Design review of the part built by this model. Coordinates are the model's own, in mm. A direction names the side the tool comes from. Coordinates: 2 decimals unless noted, no trailing zeros. Write each loop counter-clockwise with the first axis right and the second up, starting at its lowest first coordinate (ties: lowest second). Pieces come first, ordered by that corner, then holes. Notation, with made-up numbers: M -8.75,50 L -4.75,50 A23 ccw -4.75,89 Z; hole C 51,-30 d6. An arc over 180 degrees is marked long. One line per question, with ' | ' between items.
from build123d import *

# Parameters (mm, degrees)
SKETCH1_W                           = 184.15
SKETCH1_H                           = 50.8
BOSS_EXTRUDE1_DEPTH                 = 10.16
CUT_EXTRUDE1_DEPTH                  = 110.402922012
CUT_EXTRUDE1_DEPTH_BACK             = 110.402922012
SKETCH7_R                           = 22.847252038
BOSS_EXTRUDE2_DEPTH                 = 50.8
SKETCH8_R                           = 18.9865
CUT_EXTRUDE2_DEPTH                  = 45.72
SKETCH9_R                           = 7.9375
CUT_EXTRUDE3_DEPTH                  = 115.259711281
BOSS_EXTRUDE3_DEPTH                 = 50.8
BOSS_EXTRUDE4_START                 = -50.8
BOSS_EXTRUDE4_DEPTH                 = 50.8
BOSS_EXTRUDE5_START                 = -50.8
BOSS_EXTRUDE5_DEPTH                 = 50.8
CUT_EXTRUDE6_DEPTH                  = 117.385579957
F_10_CLEARANCE_HOLE1_D              = 5.1054
F_10_CLEARANCE_HOLE2_D              = 5.1054
SKETCH31_W                          = 29.960646913
SKETCH31_H                          = 50.8
BOSS_EXTRUDE6_DEPTH                 = 2.54
F_3_16_0_1875_DIAMETER_HOLE3_REACH  = 132.668
F_3_16_0_1875_DIAMETER_HOLE3_BORE_R = 2.38125
F_3_16_0_1875_DIAMETER_HOLE4_REACH  = 129.945
F_3_16_0_1875_DIAMETER_HOLE4_BORE_R = 2.38125


with BuildPart() as part:
    # Sketch1 → Boss-Extrude1 (new body)
    with BuildSketch(Plane.XY):
        with Locations((4.284398839, -3.653036721)):
            Rectangle(SKETCH1_W, SKETCH1_H)
    extrude(amount=BOSS_EXTRUDE1_DEPTH)

    # Sketch6 → Cut-Extrude1 (cut, two sides: drawn at the far end of the back side and taken through both)
    with BuildSketch(Plane(origin=(0, 21.746963279, 0), x_dir=(1, 0, 0), z_dir=(0, 1, 0)).offset(-CUT_EXTRUDE1_DEPTH_BACK)):
        with BuildLine():
            Line((189.051531618, 108.11571126), (10.888398839, 0))
            ThreePointArc((10.888398839, 0), (4.284398839, -1.847030056), (-2.319601161, 0))
            Line((-2.319601161, 0), (-180.48273394, 108.11571126))
            Line((-180.48273394, 108.11571126), (-180.48273394, 524.918345142))
            Line((-180.48273394, 524.918345142), (189.051531618, 524.918345142))
            Line((189.051531618, 524.918345142), (189.051531618, 108.11571126))
        make_face()
    extrude(amount=CUT_EXTRUDE1_DEPTH + CUT_EXTRUDE1_DEPTH_BACK, mode=Mode.SUBTRACT)

    # Sketch7 → Boss-Extrude2 (add, through all)
    with BuildSketch(Plane(origin=(0, 21.746963279, 0), x_dir=(1, 0, 0), z_dir=(0, 1, 0))):
        with Locations((4.284398839, 18.138470809)):
            Circle(SKETCH7_R)
    extrude(amount=-BOSS_EXTRUDE2_DEPTH)

    # Sketch8 → Cut-Extrude2 (cut)
    with BuildSketch(Plane(origin=(0, 21.746963279, 0), x_dir=(1, 0, 0), z_dir=(0, 1, 0))):
        with Locations(Location((4.284398839, 18.138470809, 0), (0, 0, 270))):
            Circle(SKETCH8_R)
    extrude(amount=-CUT_EXTRUDE2_DEPTH, mode=Mode.SUBTRACT)

    # Sketch9 → Cut-Extrude3 (cut, through all)
    with BuildSketch(Plane(origin=(0, -23.973036721, 0), x_dir=(1, 0, 0), z_dir=(0, 1, 0))):
        with Locations(Location((4.284398839, 18.138470809, 0), (0, 0, 270))):
            Circle(SKETCH9_R)
    extrude(amount=-CUT_EXTRUDE3_DEPTH, mode=Mode.SUBTRACT)

    # Sketch12 → Boss-Extrude3 (add)
    with BuildSketch(Plane(origin=(0, 21.746963279, 0), x_dir=(1, 0, 0), z_dir=(0, 1, 0))):
        with BuildLine():
            Line((27.131650877, 18.138470763), (27.131650877, 0))
            Line((27.131650877, 0), (18.176583779, 0))
            ThreePointArc((18.176583779, 0), (24.770920949, 8.024157287), (27.131650877, 18.138470763))
        make_face()
        with BuildLine():
            Line((-18.562853199, 18.138470775), (-18.562853199, 0))
            Line((-18.562853199, 0), (-9.607786101, 0))
            ThreePointArc((-9.607786101, 0), (-16.202123271, 8.024157294), (-18.562853199, 18.138470775))
        make_face()
    extrude(amount=-BOSS_EXTRUDE3_DEPTH)

    # Sketch16 → Boss-Extrude4 (add)
    with BuildSketch(Plane.XZ.offset(29.053036721).offset(BOSS_EXTRUDE4_START)):
        with BuildLine():
            Line((-18.562853199, -18.138470775), (-18.562853199, -40.985722847))
            Line((-18.562853199, -40.985722847), (4.284398845, -40.985722847))
            ThreePointArc((4.284398845, -40.985722847), (-11.871048017, -34.293917645), (-18.562853199, -18.138470775))
        make_face()
    extrude(amount=BOSS_EXTRUDE4_DEPTH)

    # Sketch18 → Boss-Extrude5 (add)
    with BuildSketch(Plane.XZ.offset(29.053036721).offset(BOSS_EXTRUDE5_START)):
        with BuildLine():
            Line((27.131650877, -18.138470763), (27.131650877, -40.985722847))
            Line((27.131650877, -40.985722847), (4.284398839, -40.985722847))
            ThreePointArc((4.284398839, -40.985722847), (20.439845703, -34.29391764), (27.131650877, -18.138470763))
        make_face()
    extrude(amount=BOSS_EXTRUDE5_DEPTH)

    # Sketch19 → Cut-Extrude6 (cut, through all)
    with BuildSketch(Plane(origin=(0, 21.746963279, 0), x_dir=(1, 0, 0), z_dir=(0, 1, 0))):
        Polygon((19.257650877, 40.985722847), (27.131650877, 40.985722847), (27.131650877, 33.111722847), align=None)
        Polygon((-18.562853199, 40.985722847), (-18.562853199, 33.125865684), (-10.702996036, 40.985722847), align=None)
    extrude(amount=-CUT_EXTRUDE6_DEPTH, mode=Mode.SUBTRACT)

    # #10 Clearance Hole1 (through all)
    with Locations(Plane(origin=(0, 0, 0), x_dir=(-1, 0, 0), z_dir=(0, 0, -1))):
        with Locations((78.265601161, 9.046963279), (78.265601161, -16.353036721), (-86.834398839, -16.353036721), (-86.834398839, 9.046963279)):
            Hole(F_10_CLEARANCE_HOLE1_D / 2)

    # #10 Clearance Hole2 (through all)
    with Locations(Plane(origin=(0, 0, 0), x_dir=(-1, 0, 0), z_dir=(0, 0, -1))):
        with Locations((27.465601161, -16.353036721), (27.465601161, 9.046963279), (-36.034398839, 9.046963279), (-36.034398839, -16.353036721)):
            Hole(F_10_CLEARANCE_HOLE2_D / 2)

    # Sketch31 → Boss-Extrude6 (add)
    with BuildSketch(Plane(origin=(0, 0, -40.985722847), x_dir=(-1, 0, 0), z_dir=(0, 0, -1))):
        with Locations((-4.27732742, -3.653036721)):
            Rectangle(SKETCH31_W, SKETCH31_H)
    extrude(amount=BOSS_EXTRUDE6_DEPTH)

    # 3/16 (0.1875) Diameter Hole3 bore → 3/16 (0.1875) Diameter Hole3 (cut, up to next)
    with BuildSketch(Plane(origin=(-25.844359441, 0, -25.844359441), x_dir=(-0.7071067811865462, 0, 0.7071067811865488), z_dir=(-0.7071067811865488, 0, -0.7071067811865462)), mode=Mode.PRIVATE) as f_3_16_0_1875_diameter_hole3_sk1:
        with Locations((-15.377604883, -20.163036721)):
            Circle(F_3_16_0_1875_DIAMETER_HOLE3_BORE_R)
    f_3_16_0_1875_diameter_hole3_tool1 = extrude(f_3_16_0_1875_diameter_hole3_sk1.sketch, amount=-F_3_16_0_1875_DIAMETER_HOLE3_REACH, mode=Mode.PRIVATE) & part.part
    # 3/16 (0.1875) Diameter Hole3 bore → 3/16 (0.1875) Diameter Hole3 (cut, up to next)
    with BuildSketch(Plane(origin=(-25.844359441, 0, -25.844359441), x_dir=(-0.7071067811865462, 0, 0.7071067811865488), z_dir=(-0.7071067811865488, 0, -0.7071067811865462)), mode=Mode.PRIVATE) as f_3_16_0_1875_diameter_hole3_sk2:
        with Locations((-15.377604883, -7.463036721)):
            Circle(F_3_16_0_1875_DIAMETER_HOLE3_BORE_R)
    f_3_16_0_1875_diameter_hole3_tool2 = extrude(f_3_16_0_1875_diameter_hole3_sk2.sketch, amount=-F_3_16_0_1875_DIAMETER_HOLE3_REACH, mode=Mode.PRIVATE) & part.part
    add(f_3_16_0_1875_diameter_hole3_tool1.solids().sort_by_distance((-14.970751, -20.163037, -36.717968))[0], mode=Mode.SUBTRACT)
    add(f_3_16_0_1875_diameter_hole3_tool2.solids().sort_by_distance((-14.970751, -7.463037, -36.717968))[0], mode=Mode.SUBTRACT)

    # 3/16 (0.1875) Diameter Hole4 bore → 3/16 (0.1875) Diameter Hole4 (cut, up to next)
    with BuildSketch(Plane(origin=(30.121686862, 0, -30.121686862), x_dir=(-0.7071067811865562, 0, -0.7071067811865389), z_dir=(0.7071067811865389, 0, -0.7071067811865562)), mode=Mode.PRIVATE) as f_3_16_0_1875_diameter_hole4_sk1:
        with Locations((9.308549442, -20.163036721)):
            Circle(F_3_16_0_1875_DIAMETER_HOLE4_BORE_R)
    f_3_16_0_1875_diameter_hole4_tool1 = extrude(f_3_16_0_1875_diameter_hole4_sk1.sketch, amount=-F_3_16_0_1875_DIAMETER_HOLE4_REACH, mode=Mode.PRIVATE) & part.part
    # 3/16 (0.1875) Diameter Hole4 bore → 3/16 (0.1875) Diameter Hole4 (cut, up to next)
    with BuildSketch(Plane(origin=(30.121686862, 0, -30.121686862), x_dir=(-0.7071067811865562, 0, -0.7071067811865389), z_dir=(0.7071067811865389, 0, -0.7071067811865562)), mode=Mode.PRIVATE) as f_3_16_0_1875_diameter_hole4_sk2:
        with Locations((9.308549442, -7.463036721)):
            Circle(F_3_16_0_1875_DIAMETER_HOLE4_BORE_R)
    f_3_16_0_1875_diameter_hole4_tool2 = extrude(f_3_16_0_1875_diameter_hole4_sk2.sketch, amount=-F_3_16_0_1875_DIAMETER_HOLE4_REACH, mode=Mode.PRIVATE) & part.part
    add(f_3_16_0_1875_diameter_hole4_tool1.solids().sort_by_distance((23.539548, -20.163037, -36.703825))[0], mode=Mode.SUBTRACT)
    add(f_3_16_0_1875_diameter_hole4_tool2.solids().sort_by_distance((23.539548, -7.463037, -36.703825))[0], mode=Mode.SUBTRACT)


solid = part.part
1. Take a section at D-D (z = -20). Write out the cut boundary in (x, y), then the cut area to 3 significant figures.
Answer sheet:
outline: M -18.56,-29.05 L -3.43,-29.05 L -3.43,-23.97 L -14.61,-23.97 L -14.61,21.75 L -18.56,21.75 Z; M 12,-29.05 L 27.13,-29.05 L 27.13,21.75 L 23.18,21.75 L 23.18,-23.97 L 12,-23.97 Z | area: 515 mm^2
2. To check wall thickness, follow line 1 along X through (y, z) = (14.5, -6.5); line 2 along X through (y, z) = (-13.5, -18.5); line 3 along X through (y, z) = (11, 5.5). State the ranges of each line that lie inside material, in increasing order. Write a range as [from, to].
Answer sheet:
line 1: [-18.56, -10.72], [19.29, 27.13] | line 2: [-18.56, -14.7], [23.27, 27.13] | line 3: [-87.79, -79.91], [-76.62, -29.11], [-25.82, 34.39], [37.68, 85.19], [88.48, 96.36]
3. Tool access review of faces 1 (the face through (27.132, -3, -16)), 2 (the face through (-54, -3, 0)), 3 (the face through (19.203, -8.375, -35.478)): name each direction out of +Z, -Z, +X, -X, +Y, -Y from which nothing blocks a thin tool from reaching the whole face with its end or side.
Answer sheet:
face 1: -Z, +X, +Y, -Y | face 2: -Z, -X, +Y, -Y | face 3: none
4. Take a section at B-B (z = 4). Count the separate pieces of the cut face and the enclosed holes in it, then the cut area to 3 significant figures.
Answer sheet:
separate pieces: 1 | enclosed holes: 8 | area: 9,190 mm^2
5. Insertion check: pin 1 Ø8 at (x, y) = (36.03, -16.35) entering from -Z; pin 2 Ø1.3 at (y, z) = (-16, -41.5) entering from +X; pin 3 Ø0.8 at (y, z) = (6, -43) entering from -X. Each pin has a flat end and moves straight along its axis. Give the tip position at first contact, or say it passes through.
Answer sheet:
pin 1: z = 0 | pin 2: x = 19.39 | pin 3: x = -10.7
6. Draft analysis for pull direction X (two halves, no side actions). For faces 4 (the face through (6, -29.053, -4)), 5 (the face through (-14.69, -3.3, -37)), 6 (the face through (-76.893, -14.201, 5.151)), state which applies: pulls with the +X half, pulls with the -X half, needs draft (parallel to the pull), parting line crosses it, or undercut.
Answer sheet:
face 4: needs draft | face 5: pulls with the -X half | face 6: undercut
7. Take a section at C-C (y = -12). Write out the cut boundary in (x, z).
Answer sheet:
outline: M -87.79,0 L -18.56,0 L -18.56,-33.13 L -10.7,-40.99 L -10.7,-43.53 L 19.26,-43.53 L 19.26,-40.99 L 27.13,-33.11 L 27.13,0 L 96.36,0 L 96.36,10.16 L -87.79,10.16 Z; hole C 4.28,-18.14 d37.97
8. Take a section at A-A (x = -0.5). Write out the cut boundary in (y, z).
Answer sheet:
outline: M -29.05,-43.53 L 21.75,-43.53 L 21.75,-36.51 L -23.97,-36.51 L -23.97,-24.47 L -29.05,-24.47 Z; M -29.05,-11.8 L -23.97,-11.8 L -23.97,0.24 L 21.75,0.24 L 21.75,10.16 L -29.05,10.16 Z
